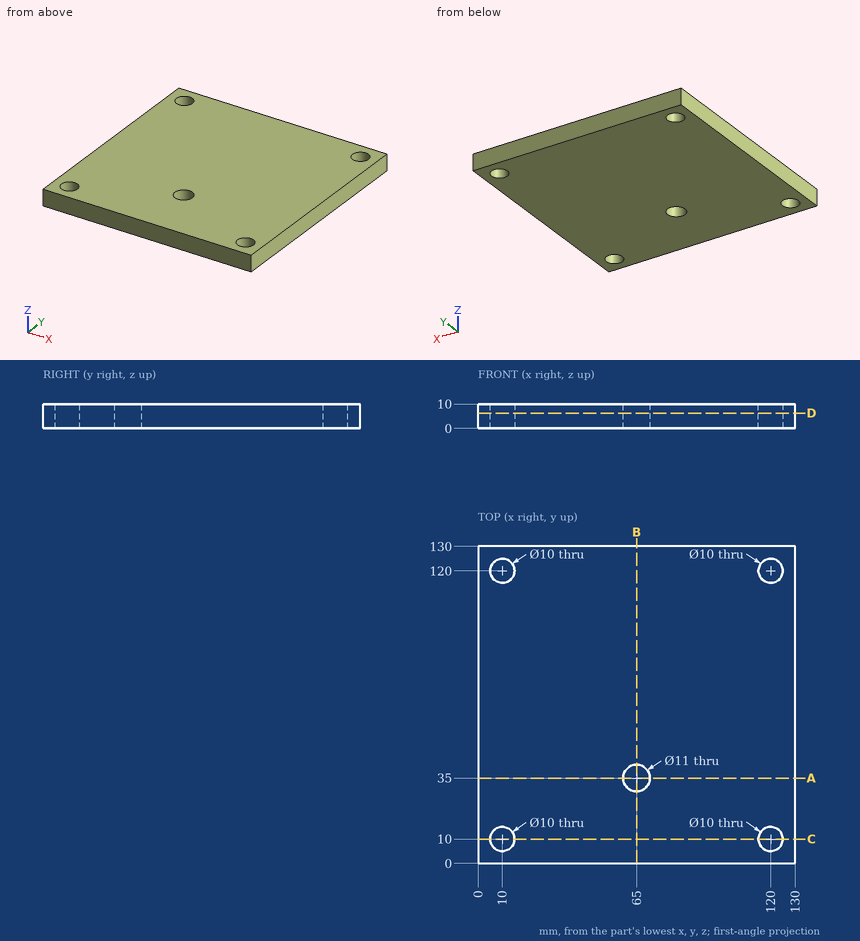
Can you work these out from the drawing? Everything is in mm from the part's minimum corner. Round coordinates to 2 decimals unless told otherwise and drop trailing zeros. Loops run counter-clockwise (first coordinate to the right, second up) from the corner with the lowest first, then second, coordinate; pieces in that order, holes last. Notation, with made-up numbers: (82, 78) - (116, 78) arc R18 cw to (116, 92) - close; hole circle Ø10 at (30.25, -22.75). An arc over 180 degrees is marked (long way). Answer in a Markdown table with one row per item. Add a question column.
Q1. I want a section at A-A on y = 35. List the corners of the cut face in (x, z) for me, and give its area (3 significant figures).
Q2. I want a section at B-B on x = 65. List the corners of the cut face in (y, z) for me.
Q3. For pin 1 Ø16 at (x, y) = (10, 120) entering from -Z; pin 2 Ø10 at (x, y) = (65, 35) entering from +Z, each with a flat end and sliding along its axis, tell me the tip position at first contact or that it passes through.
Q4. I need wall thicknesses on L1, parallel to X at y = 10, z = 6.5; L2, parallel to Y at x = 65, z = 4.75. Which ranges of each line are inside material? Lowest first, please.
Q5. I want a section at C-C on y = 10. List the corners of the cut face in (x, z) for me.
Q6. I want a section at D-D on z = 6.25. List the corners of the cut face in (x, y) for me.
A:
| question | item | result |
|---|---|---|
| 1 | outline | (0, 0) - (59.5, 0) - (59.5, 10) - (0, 10) - close; (70.5, 0) - (130, 0) - (130, 10) - (70.5, 10) - close |
| 1 | area | 1,190 mm^2 |
| 2 | outline | (0, 0) - (29.5, 0) - (29.5, 10) - (0, 10) - close; (40.5, 0) - (130, 0) - (130, 10) - (40.5, 10) - close |
| 3 | pin 1 | z = 0 |
| 3 | pin 2 | through |
| 4 | L1 | 0 to 5, 15 to 115, 125 to 130 |
| 4 | L2 | 0 to 29.5, 40.5 to 130 |
| 5 | outline | (0, 0) - (5, 0) - (5, 10) - (0, 10) - close; (15, 0) - (115, 0) - (115, 10) - (15, 10) - close; (125, 0) - (130, 0) - (130, 10) - (125, 10) - close |
| 6 | outline | (0, 0) - (130, 0) - (130, 130) - (0, 130) - close; hole circle Ø10 at (10, 10); hole circle Ø10 at (10, 120); hole circle Ø11 at (65, 35); hole circle Ø10 at (120, 10); hole circle Ø10 at (120, 120) |
